For this review, take the finished solid that the model builds, in its own axes (mm). A direction names the side the tool comes from. Give positions to 0.01 mm unless a question says otherwise; leave off trailing zeros. Write each loop counter-clockwise with the first axis right and the second up, starting at its lowest first coordinate (ties: lowest second). Pieces come first, ordered by that corner, then holes. Notation, with made-up numbers: (31, -37.75) -> (54, -37.75) arc R14 cw to (54, -16.75) -> close; hole circle Ø4 at (40, 45). An arc over 180 degrees is marked (long way). Return JSON: item names as keys, results as strings.
from build123d import *

# Parameters (mm, degrees)
F0_W     = 152.4
F0_H     = 127
F1_DEPTH = 127
F2_W     = 101.6
F2_H     = 76.2
F3_DEPTH = 76.2
F4_R     = 38.1
F5_SIZE  = 25.4
F6_W     = 50.8
F6_H     = 50.8
F7_DEPTH = 50.8
F8_R     = 25.4
F9_DEPTH = 50.801


with BuildPart() as f1:
    # F0 (on Top) → F1 (new body)
    with BuildSketch(Plane.XY):
        with Locations((19.347022, -3.683421)):
            Rectangle(F0_W, F0_H)
    extrude(amount=F1_DEPTH)

    # F2 (on face) → F3 (cut)
    with BuildSketch(Plane.XY.offset(127)):
        with Locations((44.747022, -29.083421)):
            Rectangle(F2_W, F2_H)
    extrude(amount=-F3_DEPTH, mode=Mode.SUBTRACT)

    # F4
    f4_edges = [f1.edges().sort_by_distance(p)[0] for p in [
        (-31.452978, -67.183421, 127),
    ]]
    fillet(f4_edges, radius=F4_R)

    # F5
    f5_edges = [f1.edges().sort_by_distance(p)[0] for p in [
        (95.547022, 34.416579, 127),
    ]]
    chamfer(f5_edges, length=F5_SIZE)

    # F6 (on face) → F7 (cut)
    with BuildSketch(Plane.XY.offset(127)):
        with Locations((19.347022, 34.416579)):
            Rectangle(F6_W, F6_H)
    extrude(amount=-F7_DEPTH, mode=Mode.SUBTRACT)

    # F8 (on face) → F9 (cut, through all)
    with BuildSketch(Plane.XY.offset(50.8)):
        with Locations((52.367022, -29.083421)):
            Circle(F8_R)
    extrude(amount=-F9_DEPTH, mode=Mode.SUBTRACT)


solid = f1.part
1. To check wall thickness, follow probe 1 along X at (y, z) = (5, 90); probe 2 along Z at (x, y) = (16, -19.5); probe 3 along Y at (x, z) = (62, 86). State the ranges of each line that lie inside material, in increasing order.
Results found:
{"probe 1": "x = -56.85 to -6.05", "probe 2": "z = 0 to 50.8", "probe 3": "y = 9.02 to 59.82"}
2. Add section A-A, the plane z = 78.5. State the section outline as (x, y) points, plus the area to 3 significant figures.
Results found:
{"outline": "(-56.85, -67.18) -> (-6.05, -67.18) -> (-6.05, 59.82) -> (-56.85, 59.82) -> close; (44.75, 9.02) -> (95.55, 9.02) -> (95.55, 59.82) -> (44.75, 59.82) -> close", "area": "9,030 mm²"}
3. Add section C-C, the plane y = -50.5. State the section outline as (x, z) points.
Results found:
{"outline": "(-56.85, 0) -> (38.71, 0) -> (38.71, 50.8) -> (-6.05, 50.8) -> (-6.05, 120.41) -> (-56.85, 120.41) -> close; (66.02, 0) -> (95.55, 0) -> (95.55, 50.8) -> (66.02, 50.8) -> close"}
4. For pin 1 (23 mm diameter, centred on x = 46, z = 92.5, fed in from -Y); pin 2 (15 mm diameter, centred on x = 16.5, y = 38, fed in from +Z); pin 3 (2 mm diameter, centred on y = -34, z = 63.5, fed in from +X), all flat-tipped, find the tip position at first contact; note any pin that passes through.
Results found:
{"pin 1": "stops at y = 9.02", "pin 2": "stops at z = 76.2", "pin 3": "stops at x = -6.05"}
5. For faces 4 (the flat face through (44.747, 34, 102)), 5 (the flat face through (55, 9.017, 81)), 6 (the flat face through (-6.053, -5, 89)), list the 3-axis set-ups (+Z, -Z, +X, -X, +Y, -Y) from which the entire face can be reached by the end or side of a thin tool; tool diameter is ignored.
Results found:
{"face 4": "+Z, +Y, -Y", "face 5": "+Z, +X, -Y", "face 6": "+Z, -Y"}
6. The part is to be moulded in two halves that separate along Y. For faces 1 (the cylindrical face through (-31.1, -56.32, 115.54)), 2 (the cylindrical face through (26.99, -27.97, 25.76)), 3 (the flat face through (19, 35, 76.2)), say which applies: +Y half, -Y half, draft (parallel to the pull), parting line (faces both ways), or undercut.
Results found:
{"face 1": "-Y half", "face 2": "undercut", "face 3": "draft"}
7. Add section D-D, the plane z = 41.5. State the section outline as (x, y) points.
Results found:
{"outline": "(-56.85, -67.18) -> (95.55, -67.18) -> (95.55, 59.82) -> (-56.85, 59.82) -> close; hole circle Ø50.8 at (52.37, -29.08)"}
8. Add section B-B, the plane x = 66.5. State the section outline as (y, z) points, plus the area to 3 significant figures.
Results found:
{"outline": "(-67.18, 0) -> (-50.19, 0) -> (-50.19, 50.8) -> (-67.18, 50.8) -> close; (-7.98, 0) -> (59.82, 0) -> (59.82, 127) -> (9.02, 127) -> (9.02, 50.8) -> (-7.98, 50.8) -> close", "area": "8,180 mm²"}
